```python
from build123d import *

# Parameters (mm, degrees)
SKETCH_1_R          = 2.6
EXTRUDE_1_DEPTH     = 3
SKETCH_2_W          = 36
SKETCH_2_H          = 36
EXTRUDE_2_DEPTH     = 3
CUT_EXTRUDE_1_REACH = 43.827
SKETCH_3_R          = 1.6
CUT_EXTRUDE_2_DEPTH = 3
FILLET_1_R          = 1
FILLET_2_R          = 10


with BuildPart() as part:
    # 草图1 → 凸台-拉伸1 (new body)
    # profile 1 of 5: a face of its own
    with BuildSketch(Plane.XY):
        with BuildLine():
            Line((-28.181980515, 21.818019485), (-6.363961031, 0))
            Line((-6.363961031, 0), (0, 6.363961031))
            Line((0, 6.363961031), (-21.818019485, 28.181980515))
            ThreePointArc((-21.818019485, 28.181980515), (-28.181980515, 28.181980515), (-28.181980515, 21.818019485))
        make_face()
        with Locations((-25, 25)):
            Circle(SKETCH_1_R, mode=Mode.SUBTRACT)
    # profile 2 of 5: a face of its own
    with BuildSketch(Plane.XY):
        with BuildLine():
            Line((-6.363961031, 0), (-28.181980515, -21.818019485))
            ThreePointArc((-28.181980515, -21.818019485), (-28.181980515, -28.181980515), (-21.818019485, -28.181980515))
            Line((-21.818019485, -28.181980515), (0, -6.363961031))
            Line((0, -6.363961031), (-6.363961031, 0))
        make_face()
        with Locations((-25, -25)):
            Circle(SKETCH_1_R, mode=Mode.SUBTRACT)
    # profile 3 of 5: a face of its own
    with BuildSketch(Plane.XY):
        with BuildLine():
            Line((6.363961031, 0), (0, -6.363961031))
            Line((0, -6.363961031), (21.818019485, -28.181980515))
            ThreePointArc((21.818019485, -28.181980515), (28.181980515, -28.181980515), (28.181980515, -21.818019485))
            Line((28.181980515, -21.818019485), (6.363961031, 0))
        make_face()
        with Locations((25, -25)):
            Circle(SKETCH_1_R, mode=Mode.SUBTRACT)
    # profile 4 of 5: a face of its own
    with BuildSketch(Plane.XY):
        with BuildLine():
            Line((21.818019485, 28.181980515), (0, 6.363961031))
            Line((0, 6.363961031), (6.363961031, 0))
            Line((6.363961031, 0), (28.181980515, 21.818019485))
            ThreePointArc((28.181980515, 21.818019485), (28.181980515, 28.181980515), (21.818019485, 28.181980515))
        make_face()
        with Locations((25, 25)):
            Circle(SKETCH_1_R, mode=Mode.SUBTRACT)
    # profile 5 of 5: a face of its own
    with BuildSketch(Plane.XY):
        Polygon((0, 6.363961031), (-6.363961031, 0), (0, -6.363961031), (6.363961031, 0), align=None)
    extrude(amount=EXTRUDE_1_DEPTH)

    # 草图2 → 凸台-拉伸2 (add)
    with BuildSketch(Plane.XY.offset(3)):
        Rectangle(SKETCH_2_W, SKETCH_2_H)
    extrude(amount=-EXTRUDE_2_DEPTH)

    # 草图3 → 切除-拉伸1 (cut, up to next)
    with BuildSketch(Plane.XY.offset(3), mode=Mode.PRIVATE) as cut_extrude_1_sk1:
        with Locations((0, -12.5)):
            Circle(SKETCH_3_R)
    cut_extrude_1_tool1 = extrude(cut_extrude_1_sk1.sketch, amount=-CUT_EXTRUDE_1_REACH, mode=Mode.PRIVATE) & part.part
    # 草图3 → 切除-拉伸1 (cut, up to next)
    with BuildSketch(Plane.XY.offset(3), mode=Mode.PRIVATE) as cut_extrude_1_sk2:
        with Locations((0, 12.5)):
            Circle(SKETCH_3_R)
    cut_extrude_1_tool2 = extrude(cut_extrude_1_sk2.sketch, amount=-CUT_EXTRUDE_1_REACH, mode=Mode.PRIVATE) & part.part
    # 草图3 → 切除-拉伸1 (cut, up to next)
    with BuildSketch(Plane.XY.offset(3), mode=Mode.PRIVATE) as cut_extrude_1_sk3:
        with Locations((4.783542905, 11.548494156)):
            Circle(SKETCH_3_R)
    cut_extrude_1_tool3 = extrude(cut_extrude_1_sk3.sketch, amount=-CUT_EXTRUDE_1_REACH, mode=Mode.PRIVATE) & part.part
    # 草图3 → 切除-拉伸1 (cut, up to next)
    with BuildSketch(Plane.XY.offset(3), mode=Mode.PRIVATE) as cut_extrude_1_sk4:
        with Locations((-4.783542905, -11.548494156)):
            Circle(SKETCH_3_R)
    cut_extrude_1_tool4 = extrude(cut_extrude_1_sk4.sketch, amount=-CUT_EXTRUDE_1_REACH, mode=Mode.PRIVATE) & part.part
    # 草图3 → 切除-拉伸1 (cut, up to next)
    with BuildSketch(Plane.XY.offset(3), mode=Mode.PRIVATE) as cut_extrude_1_sk5:
        with Locations((4.783542905, -11.548494156)):
            Circle(SKETCH_3_R)
    cut_extrude_1_tool5 = extrude(cut_extrude_1_sk5.sketch, amount=-CUT_EXTRUDE_1_REACH, mode=Mode.PRIVATE) & part.part
    # 草图3 → 切除-拉伸1 (cut, up to next)
    with BuildSketch(Plane.XY.offset(3), mode=Mode.PRIVATE) as cut_extrude_1_sk6:
        with Locations((-4.783542905, 11.548494156)):
            Circle(SKETCH_3_R)
    cut_extrude_1_tool6 = extrude(cut_extrude_1_sk6.sketch, amount=-CUT_EXTRUDE_1_REACH, mode=Mode.PRIVATE) & part.part
    add(cut_extrude_1_tool1.solids().sort_by_distance((0, -12.5, 3))[0], mode=Mode.SUBTRACT)
    add(cut_extrude_1_tool2.solids().sort_by_distance((0, 12.5, 3))[0], mode=Mode.SUBTRACT)
    add(cut_extrude_1_tool3.solids().sort_by_distance((4.783543, 11.548494, 3))[0], mode=Mode.SUBTRACT)
    add(cut_extrude_1_tool4.solids().sort_by_distance((-4.783543, -11.548494, 3))[0], mode=Mode.SUBTRACT)
    add(cut_extrude_1_tool5.solids().sort_by_distance((4.783543, -11.548494, 3))[0], mode=Mode.SUBTRACT)
    add(cut_extrude_1_tool6.solids().sort_by_distance((-4.783543, 11.548494, 3))[0], mode=Mode.SUBTRACT)

    # 草图4 → 切除-拉伸2 (cut)
    with BuildSketch(Plane.XY.offset(3)):
        Polygon((14, -15.556766946), (14, 15.556766946), (1.900292375, 0), align=None)
        Polygon((-14, -15.556766946), (-1.900292375, 0), (-14, 15.556766946), align=None)
    extrude(amount=-CUT_EXTRUDE_2_DEPTH, mode=Mode.SUBTRACT)

    # 圆角1
    fillet_1_edges = [part.edges().sort_by_distance(p)[0] for p in [
        (14, 15.556766946, 1.5),
        (14, -15.556766946, 1.5),
        (1.900292375, 0, 1.5),
        (-14, -15.556766946, 1.5),
        (-14, 15.556766946, 1.5),
        (-1.900292375, 0, 1.5),
    ]]
    fillet(fillet_1_edges, radius=FILLET_1_R)

    # 圆角2
    fillet_2_edges = [part.edges().sort_by_distance(p)[0] for p in [
        (18, -11.636038969, 1.5),
        (-11.636038969, -18, 1.5),
        (-18, -11.636038969, 1.5),
        (18, 11.636038969, 1.5),
        (11.636038969, -18, 1.5),
        (-18, 11.636038969, 1.5),
        (-11.636038969, 18, 1.5),
        (11.636038969, 18, 1.5),
    ]]
    fillet(fillet_2_edges, radius=FILLET_2_R)


solid = part.part
```
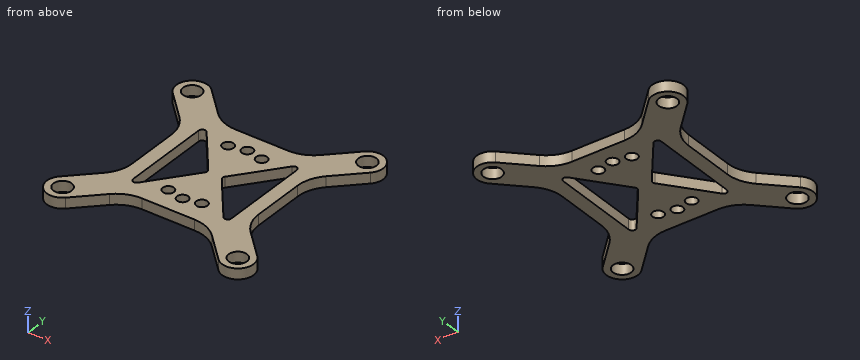
Input: part model. Units: mm. Frame: model coordinates. Round coordinates to 2 decimals unless told otherwise and drop trailing zeros. Loops run counter-clockwise (first coordinate to the right, second up) from the corner with the lowest first, then second, coordinate; pieces in that order, holes last. Notation, with made-up numbers: M -22.5,1 L 14.5,1 A32 ccw 14.5,29 Z; hole C 20.25,88 d1. An arc over 180 degrees is marked long. Answer in a Markdown table with one row per item. Add a question column.
1. Ray query, probe 1 along Y at (x, z) = (0, 2.05); probe 2 along X at (y, z) = (7, 0.55); probe 3 along Y at (x, z) = (-25, 1.75). Return the intervals inside material, ascending.
2. Section B-B (y = -9). Output: boundary loops of the cut face in (x, z), and give its area (3 significant figures).
3. Contact query for flat-ended pins moving along their axis: pin 1 (1.5 mm diameter, centred on y = -1.5, z = 1.5, fed in from +X); pin 2 (3.5 mm diameter, centred on x = -4.78, y = 11.55, fed in from +Z); pin 3 (1.5 mm diameter, centred on y = 3, z = 2, fed in from -X); pin 4 (1 mm diameter, centred on x = 7, z = 1.5, fed in from +Y). Output: stop coordinate, or through.
4. Section C-C (y = -25). Output: boundary loops of the cut face in (x, z).
5. Section D-D (x = 9). Output: boundary loops of the cut face in (y, z).
6. Section A-A (x = 0). Output: boundary loops of the cut face in (y, z), and give its area (3 significant figures).
Values follow:
| question | item | result |
|---|---|---|
| 1 | probe 1 | -18 to -14.1, -10.9 to 10.9, 14.1 to 18 |
| 1 | probe 2 | -18 to -14, -7.34 to 7.34, 14 to 18 |
| 1 | probe 3 | -29.5 to -27.6, -22.4 to -18.64, 18.64 to 22.4, 27.6 to 29.5 |
| 2 | outline | M -18.11,0 L -14,0 L -14,3 L -18.11,3 Z; M -8.9,0 L 8.9,0 L 8.9,3 L -8.9,3 Z; M 14,0 L 18.11,0 L 18.11,3 L 14,3 Z |
| 2 | area | 78.1 mm^2 |
| 3 | pin 1 | x = 18 |
| 3 | pin 2 | z = 3 |
| 3 | pin 3 | x = -18 |
| 3 | pin 4 | y = 18 |
| 4 | outline | M -29.5,0 L -27.6,0 L -27.6,3 L -29.5,3 Z; M -22.4,0 L -18.64,0 L -18.64,3 L -22.4,3 Z; M 18.64,0 L 22.4,0 L 22.4,3 L 18.64,3 Z; M 27.6,0 L 29.5,0 L 29.5,3 L 27.6,3 Z |
| 5 | outline | M -18.11,0 L -9.13,0 L -9.13,3 L -18.11,3 Z; M 9.13,0 L 18.11,0 L 18.11,3 L 9.13,3 Z |
| 6 | outline | M -18,0 L -14.1,0 L -14.1,3 L -18,3 Z; M -10.9,0 L 10.9,0 L 10.9,3 L -10.9,3 Z; M 14.1,0 L 18,0 L 18,3 L 14.1,3 Z |
| 6 | area | 88.8 mm^2 |
